Autodesk Inventor part; units mm, degrees
ref_plane "Work Plane1" through (-0.635, 46.99, -50.8) normal (0, 1, 0) x (0, 0, 1)
ref_plane "YZ Plane" through (0, 0, 0) normal (1, 0, 0) x (0, 1, 0)
ref_plane "XZ Plane" through (0, 0, 0) normal (0, 1, 0) x (-1, 0, 0)
sketch "Sketch1" plane through (0, 0, 0) normal (0, 0, 1) x (1, 0, 0)
  line L0 (7.62, 0) -> (62.23, 0)
  line L1 (69.85, 7.62) -> (69.85, 36.83)
  line L2 (62.23, 44.45) -> (7.62, 44.45)
  line L3 (0, 36.83) -> (0, 7.62)
  arc A0 (7.62, 44.45) -> (0, 36.83) centre (7.62, 36.83) ccw
  arc A1 (0, 7.62) -> (7.62, 0) centre (7.62, 7.62) ccw
  arc A2 (62.23, 0) -> (69.85, 7.62) centre (62.23, 7.62) ccw
  arc A3 (69.85, 36.83) -> (62.23, 44.45) centre (62.23, 36.83) ccw
  point P0 (0, 0)
  point P1 (69.85, 44.45)
  point P2 (69.85, 0)
  point P3 (0, 44.45)
  dimension "d0" = 69.85
  dimension "d1" = 44.45
  dimension "d2" = 7.62
extrude "Extrusion1" add sketch "Sketch1" along normal blind 9
sketch "Sketch2" plane through (0, 0, 9) normal (0, 0, 1) x (1, 0, 0)
  line L0 (4.445, -3.175) -> (65.405, -3.175)
  line L1 (73.025, 4.445) -> (73.025, 40.005)
  line L2 (65.405, 47.625) -> (4.445, 47.625)
  line L3 (-3.175, 40.005) -> (-3.175, 4.445)
  arc A0 (4.445, 47.625) -> (-3.175, 40.005) centre (4.445, 40.005) ccw
  arc A1 (-3.175, 4.445) -> (4.445, -3.175) centre (4.445, 4.445) ccw
  arc A2 (65.405, -3.175) -> (73.025, 4.445) centre (65.405, 4.445) ccw
  arc A3 (73.025, 40.005) -> (65.405, 47.625) centre (65.405, 40.005) ccw
  line L4 (62.23, 44.45) -> (7.62, 44.45) construction
  line L5 (0, 36.83) -> (0, 7.62) construction
  point P0 (0, 0)
  point P1 (73.025, 47.625)
  point P2 (73.025, -3.175)
  point P3 (-3.175, 47.625)
  point P4 (34.925, 47.625)
  point P5 (34.925, 44.45)
  point P6 (-3.175, 22.225)
  point P7 (0, 22.225)
  dimension "d5" = 76.2
  dimension "d6" = 50.8
  dimension "d7" = 7.62
extrude "Extrusion2" add sketch "Sketch2" along normal blind 12.7
fillet "Fillet1" [suppressed]
sketch "Sketch3" plane through (0, 0, 21.7) normal (0, 0, 1) x (1, 0, 0)
  line L0 (65.405, 47.625) -> (4.445, 47.625) construction
  line L1 (65.405, 47.625) -> (4.445, 47.625) construction
  line L2 (-3.175, 40.005) -> (-3.175, 4.445) construction
  line L3 (-3.175, 40.005) -> (-3.175, 4.445) construction
  circle A0 centre (34.925, 22.225) radius 8.75
  circle A1 centre (34.925, 22.225) radius 19 construction
  circle A2 centre (21.49, 35.66) radius 2.25
  circle A3 centre (48.36, 35.66) radius 2.25
  circle A4 centre (15.925, 22.225) radius 2.25
  circle A5 centre (53.925, 22.225) radius 2.25
  circle A6 centre (21.49, 8.79) radius 2.25
  circle A7 centre (48.36, 8.79) radius 2.25
  line L4 (21.49, 35.66) -> (34.925, 22.225) construction
  line L5 (34.925, 22.225) -> (15.925, 22.225) construction
  point P0 (0, 0)
  point P1 (34.925, 47.625)
  point P2 (-3.175, 22.225)
  point P3 (-3.175, 22.225)
  dimension "d11" = 17.5
  dimension "d14" = 4.5
  dimension "d15" = 38
  dimension "d16" = 45
extrude "Extrusion3" cut sketch "Sketch3" against normal up to surface (21.7 mm away)
chamfer "Chamfer1" distance 1.27 angle 45 6 edges at (46.11, 35.66, 0) (19.24, 35.66, 0) (13.675, 22.225, 0) (51.675, 22.225, 0) (46.11, 8.79, 0) (19.24, 8.79, 0)
sketch "Sketch4" plane through (7.62, 0, 0) normal (0, -1, 0) x (1, 0, 0)
  point P0 (-7.62, 0)
ref_plane "Work Plane1" through (-0.635, 46.99, -50.8) normal (0, 1, 0) x (0, 0, 1)
sketch "Sketch8" plane through (0, 0, 0) normal (0, 0, -1) x (-1, 0, 0)
  point P0 (0, 0)
fillet "Fillet2" radius 0.635 1 edges at (26.175, 22.225, 0)
properties part number "2x3_Spacer_Rear_metal"
Could you check a few things on this model? Use its own coordinates, in mm. A direction names the side the tool comes from. Give positions to 0.01 mm unless a question says otherwise; leave off trailing zeros. Write each loop counter-clockwise with the first axis right and the second up, starting at its lowest first coordinate (ties: lowest second). Pieces come first, ordered by that corner, then holes. Notation, with made-up numbers: (33.5, 42) -> (72.5, 42) arc R23 ccw to (72.5, 72) -> close; hole circle Ø11 at (53, 22.5). An arc over 180 degrees is marked (long way). Answer as a JSON object with one key per item and string values.
Q1. Will these pins go through, and if not, where does the flat tip stop? pin 1 Ø10 at (y, z) = (19, 2.5) entering from -X; pin 2 Ø2 at (x, y) = (53, 14) entering from -Z; pin 3 Ø7 at (x, z) = (25.5, 2.5) entering from -Y; pin 4 Ø4.5 at (x, z) = (27, 4) entering from +Y.
Taken from the geometry:
{"pin 1": "stops at x = 0", "pin 2": "stops at z = 0", "pin 3": "stops at y = 0", "pin 4": "stops at y = 44.45"}
Q2. Suppose I cut it at A-A on x = 48.36. Write out the boundary of the cut face in (y, z) (3 decimals).
Taken from the geometry:
{"outline": "(-3.175, 9) -> (0, 9) -> (0, 0) -> (5.27, 0) -> (6.54, 1.27) -> (6.54, 21.7) -> (-3.175, 21.7) -> close; (11.04, 1.27) -> (12.31, 0) -> (32.14, 0) -> (33.41, 1.27) -> (33.41, 21.7) -> (11.04, 21.7) -> close; (37.91, 1.27) -> (39.18, 0) -> (44.45, 0) -> (44.45, 9) -> (47.625, 9) -> (47.625, 21.7) -> (37.91, 21.7) -> close"}
Q3. Which directions (+Z, -Z, +X, -X, +Y, -Y) give clear straight access to the entire face, cutting with the end or side of a thin tool? Please do faces 1 (the flat face through (35, 44.45, 4)), 2 (the flat face through (35, 0, 4)), 3 (the flat face through (69.85, 22, 4)), 4 (the cylindrical face through (67.677, 2.291, 4.437)).
Taken from the geometry:
{"face 1": "-Z, +X, -X, +Y", "face 2": "-Z, +X, -X, -Y", "face 3": "-Z, +X, +Y, -Y", "face 4": "-Z, +X, -Y"}
Q4. Suppose I cut it at D-D on x = 10. Write out the boundary of the cut face in (y, z) (3 decimals).
Taken from the geometry:
{"outline": "(-3.175, 9) -> (0, 9) -> (0, 0) -> (44.45, 0) -> (44.45, 9) -> (47.625, 9) -> (47.625, 21.7) -> (-3.175, 21.7) -> close"}
Q5. Suppose I cut it at B-B on y = 35.66. Write out the boundary of the cut face in (x, z) (3 decimals), then the cut area to 3 significant figures.
Taken from the geometry:
{"outline": "(-3.175, 9) -> (0, 9) -> (0, 0) -> (17.97, 0) -> (19.24, 1.27) -> (19.24, 21.7) -> (-3.175, 21.7) -> close; (23.74, 1.27) -> (25.01, 0) -> (44.84, 0) -> (46.11, 1.27) -> (46.11, 21.7) -> (23.74, 21.7) -> close; (50.61, 1.27) -> (51.88, 0) -> (69.85, 0) -> (69.85, 9) -> (73.025, 9) -> (73.025, 21.7) -> (50.61, 21.7) -> close", "area": "1,400 mm²"}
Q6. Suppose I cut it at C-C on z = 18.25. Write out the boundary of the cut face in (x, y) (3 decimals).
Taken from the geometry:
{"outline": "(-3.175, 4.445) arc R7.62 ccw to (4.445, -3.175) -> (65.405, -3.175) arc R7.62 ccw to (73.025, 4.445) -> (73.025, 40.005) arc R7.62 ccw to (65.405, 47.625) -> (4.445, 47.625) arc R7.62 ccw to (-3.175, 40.005) -> close; hole circle Ø4.5 at (15.925, 22.225); hole circle Ø4.5 at (21.49, 8.79); hole circle Ø4.5 at (21.49, 35.66); hole circle Ø17.5 at (34.925, 22.225); hole circle Ø4.5 at (48.36, 8.79); hole circle Ø4.5 at (48.36, 35.66); hole circle Ø4.5 at (53.925, 22.225)"}
Q7. We'd pull the mould along X, two halves only. Please class faces 5 (the flat face through (26, 23, 21.7)), 6 (the cylindrical face through (23.636, 9.466, 11.628)), 7 (the flat face through (-3.175, 22, 15)): released by +X, released by -X, zero draft, split by the parting line, or undercut.
Taken from the geometry:
{"face 5": "zero draft", "face 6": "undercut", "face 7": "released by -X"}
Q8. Please list where these lines run through material, in increasing order: L1, parallel to Y at x = 21.49, z = 6.25; L2, parallel to Y at x = 47, z = 13.5 (3 decimals); L3, parallel to X at y = 23, z = 8.5.
Taken from the geometry:
{"L1": "y = 0 to 6.54, 11.04 to 33.41, 37.91 to 44.45", "L2": "y = -3.175 to 6.998, 10.582 to 33.868, 37.452 to 47.625", "L3": "x = 0 to 13.81, 18.04 to 26.21, 43.64 to 51.81, 56.04 to 69.85"}
